Autodesk Inventor part; units mm, degrees
ref_plane "YZ Plane" through (0, 0, 0) normal (1, 0, 0) x (0, 1, 0)
ref_plane "XZ Plane" through (0, 0, 0) normal (0, 1, 0) x (-1, 0, 0)
sketch "Sketch1" plane through (0, 0, 0) normal (0, 1, 0) x (-1, 0, 0)
  circle A0 centre (0, 0) radius 20.32
  circle A1 centre (0, 0) radius 16.7005
  dimension "d0" = 40.64
  dimension "d1" = 33.401
extrude "Extrusion1" add sketch "Sketch1" along normal blind 79.0448
ref_plane "Work Plane1" through (0, 0, 20.32) normal (0, 0, 1) x (1, 0, 0)
sketch "Sketch2" plane through (0, 0, 20.32) normal (0, 0, 1) x (1, 0, 0)
  line L0 (0, 0) -> (0, 79.0448)
  line L1 (20.32, 79.0448) -> (-20.32, 79.0448)
  line L2 (-20.32, 0) -> (-20.32, 79.0448)
  line L3 (-20.32, 39.5224) -> (20.32, 39.5224)
  line L4 (20.32, 0) -> (20.32, 79.0448)
  circle A0 centre (0, 39.5224) radius 16.7005
  circle A1 centre (0, 39.5224) radius 20.32
  dimension "d4" = 33.401
  dimension "d5" = 40.64
extrude "Extrusion2" add sketch "Sketch2" along normal blind 16.51 and the other way blind 8.255 contours A1 L3 A0 L0 | L0 A0 L3 A1 | A1 L0 A0 L3 | L3 A0 L0 A1
sketch "Sketch3" plane through (0, 39.5224, 36.83) normal (0, 0, 1) x (1, 0, 0)
  circle A0 centre (0, 0) radius 16.7005
  point P0 (0, -39.5224)
  dimension "d10" = 33.401
extrude "Extrusion3" cut sketch "Sketch3" against normal blind 25.4
properties part number "New Elbow"
Verification items for the finished model (mm, model axes). A direction names the side the tool comes from. Round coordinates to 2 decimals unless told otherwise and drop trailing zeros. Order: outer loops, then holes, each group sorted by start corner. A loop starts at its lowest first (then second) coordinate and runs counter-clockwise, first axis right, second up.
1) Material ranges on line 1 (Z direction, x = 0, y = 22) (1 decimal); line 2 (Y direction, x = 0, z = 18); line 3 (Y direction, x = 0, z = 23.75), recorded low to high.
Geometry says:
line 1: z = -20.3 to -16.7, 12.1 to 36.8
line 2: y = 0 to 22.82, 56.22 to 79.04
line 3: y = 19.2 to 22.82, 56.22 to 59.84
2) Cross-section at B-B, the plane x = 0. Record the cut outline in (y, z) (1 decimal).
Geometry says:
outline: (0, -20.3) - (79, -20.3) - (79, -16.7) - (0, -16.7) - close; (0, 16.7) - (19.2, 16.7) - (19.2, 12.1) - (22.8, 12.1) - (22.8, 36.8) - (19.2, 36.8) - (19.2, 20.3) - (0, 20.3) - close; (56.2, 12.1) - (59.8, 12.1) - (59.8, 16.7) - (79, 16.7) - (79, 20.3) - (59.8, 20.3) - (59.8, 36.8) - (56.2, 36.8) - close
3) Draft check along Y on faces 1 (the cylindrical face through (2.17, 38.97, -16.56)), 2 (the flat face through (14, 40, 11.43)), 3 (the cylindrical face through (-4.405, 19.686, 27.373)), 4 (the cylindrical face through (8.978, 53.604, 24.308)). Enter one of: +Y half, -Y half, draft (parallel to the pull), parting line (faces both ways), or undercut.
Geometry says:
face 1: draft
face 2: undercut
face 3: parting line
face 4: undercut
4) Tool access check on faces 5 (the flat face through (2, 0, 17)), 6 (the flat face through (0, 22, 12.065)), 7 (the flat face through (-14, 40, 11.43)). Record the directions out of +Z, -Z, +X, -X, +Y, -Y that give a thin tool (end or side, any length) a straight path to the whole face; none if there is none.
Geometry says:
face 5: +Z, -Z, +X, -X, -Y
face 6: +Y, -Y
face 7: +Z
5) Cross-section at D-D, the plane y = 49.5. Record the cut outline in (x, z) (1 decimal).
Geometry says:
outline: (-17.7, 12.1) - (-16.4, 12.1) arc R20.3 ccw (long way) to (16.4, 12.1) - (17.7, 12.1) - (17.7, 36.8) - (13.4, 36.8) - (13.4, 11.4) - (12.2, 11.4) arc R16.7 cw (long way) to (-12.2, 11.4) - (-13.4, 11.4) - (-13.4, 36.8) - (-17.7, 36.8) - close
6) Cross-section at C-C, the plane x = -14.5. Record the cut outline in (y, z).
Geometry says:
outline: (0, -14.24) - (79.04, -14.24) - (79.04, -8.29) - (0, -8.29) - close; (0, 8.29) - (79.04, 8.29) - (79.04, 14.24) - (53.76, 14.24) - (53.76, 36.83) - (47.81, 36.83) - (47.81, 11.43) - (31.24, 11.43) - (31.24, 36.83) - (25.29, 36.83) - (25.29, 14.24) - (0, 14.24) - close
7) Depth check by flat-ended pin: pin 1 (4 mm diameter, centred on x = -3.5, y = 70, fed in from -Z); pin 2 (5 mm diameter, centred on x = 15.5, z = 31, fed in from -Y) (3 decimals); pin 3 (12 mm diameter, centred on x = -8, y = 59, fed in from -Z). Enter the tip coordinate at first touch or a pass-through.
Geometry says:
pin 1: stops at z = -20.26
pin 2: stops at y = 23.905
pin 3: stops at z = -20.22
8) Cross-section at A-A, the plane z = 0. Record the cut outline in (x, y).
Geometry says:
outline: (-20.32, 0) - (-16.7, 0) - (-16.7, 79.04) - (-20.32, 79.04) - close; (16.7, 0) - (20.32, 0) - (20.32, 79.04) - (16.7, 79.04) - close
